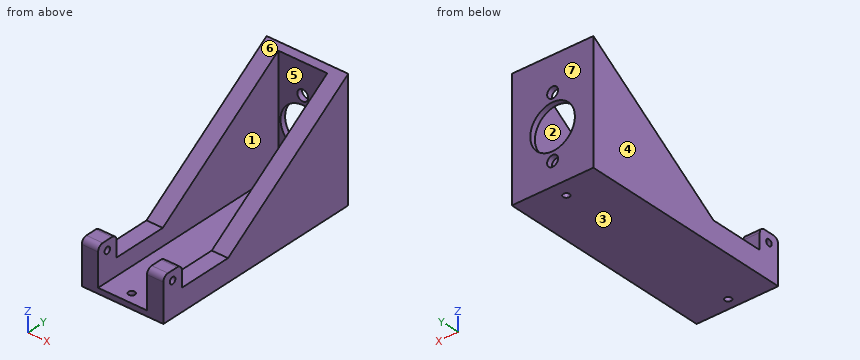
Solid Edge part; units mm, degrees
sketch "Sketch1" plane through (0, 0, 0) normal (0, -1, 0) x (1, 0, 0)
  line L0 (0, 110) -> (0, 0)
  line L1 (0, 0) -> (75, 0)
  line L2 (75, 0) -> (75, 110)
  line L3 (75, 110) -> (0, 110)
  dimension "D1" = 75
extrude "Protrusion1" add sketch "Sketch1" against normal blind 200
sketch "Sketch2" plane through (37.5, 0, 62.5) normal (0, -1, 0) x (1, 0, 0)
  line L0 (-22.5, 47.5) -> (-22.5, -57.5)
  line L1 (-22.5, -57.5) -> (22.5, -57.5)
  line L2 (22.5, -57.5) -> (22.5, 47.5)
  dimension "D1" = 22.5
extrude "ExtrudedCutout_1" cut sketch "Sketch2" against normal blind 195 material side at (15.05, 0, 57.5)
sketch "Sketch3" plane through (0, 100, 62.5) normal (-1, 0, 0) x (0, -1, 0)
  line L0 (-100, 47.5) -> (30, -42.1258)
  line L1 (30, -42.1258) -> (80, -42.1258)
  line L2 (80, -42.1258) -> (80, -22.5)
  line L3 (80, -22.5) -> (100, -22.5)
  line L4 (100, 47.5) -> (100, -22.5)
  line L5 (-100, 47.5) -> (100, 47.5)
  dimension "D1" = 80
  dimension "D2" = 30
  dimension "D3" = 100
extrude "ExtrudedCutout_2" cut sketch "Sketch3" against normal blind 140
hole "hål_till_pedal_vänster" at (0, 10, 31.4) direction (1, 0, 0) diameter 6 end up to next
hole "Hål_till_pedal_höger_" at (75, 10, 31.4) direction (-1, 0, 0) diameter 6 end up to next
fillet "Avrundning" radius 5 4 edges at (67.5, 0, 40) (67.5, 20, 40) (7.5, 0, 40) (7.5, 20, 40)
hole "Hål_till_huvudcylinder" at (37.5, 200, 50) direction (0, -1, 0) diameter 41 end up to next
hole "Hole1" at (37.5, 200, 78.6) direction (0, -1, 0) diameter 10 end up to next
hole "Hole2" at (37.5, 200, 21.4) direction (0, -1, 0) diameter 10 end up to next
hole "Hole3" at (37.5, 10, 5) direction (0, 0, -1) diameter 6 end through all
hole "Hole4" at (37.5, 185, 5) direction (0, 0, -1) diameter 6 end through all
properties material "Aluminum, 1060"
Geometry: final body of the model. Coordinates: model frame, mm. Face numbers are marked on the shaded views. A direction names the side the tool comes from. Coordinates: 2 decimals unless noted, no trailing zeros. Order: outer loops, then holes, each group sorted by start corner. A loop starts at its lowest first (then second) coordinate and runs counter-clockwise, first axis right, second up. Notation, with made-up numbers: M 46.5,44 L 97.5,44 A9 cw 97.5,50 Z; hole C 28.5,30.25 d4. An arc over 180 degrees is marked long. Answer in a Markdown table with one row per item. Add a question column.
Q1. Mould query, pull axis X, two halves, no side actions, for the marked faces 1, 2, 3 and 4. Classes: released by +X, released by -X, zero draft, split by the parting line, or undercut.
Q2. Line query: L1, parallel to Y at x = 37, z = 2; L2, parallel to Z at x = 65, y = 10; L3, parallel to X at y = 160, z = 37. Output: solid intervals per line, ascending.
Q3. Section query B-B on x = 64. Return the cut outline in (y, z).
Q4. Reachability of the marked faces 5, 6 and 7 from +Z, -Z, +X, -X, +Y, -Y: full face, straight path, thin tool, end or side. Return the list, or none.
Q5. Contact query for flat-ended pins moving along their axis: P1, Ø12, axis at y = 74, z = 29.5, coming from the +X side; P2, Ø12, axis at x = 67.5, y = 34, coming from the +Z side; P3, Ø5, axis at x = 4.5, y = 8.5, coming from the +Z side; P4, Ø22.5, axis at x = 29, y = 86.5, coming from the +Z side. Output: stop coordinate, or through.
Q6. Section query A-A on x = 37.5. Return the cut outline in (y, z), and give its area (3 significant figures).
Q7. Section query D-D on z = 45. Return the cut outline in (x, y), and give its area (3 significant figures).
Q8. Section query C-C on y = 10. Return the cut outline in (x, z).
Completed:
| question | item | result |
|---|---|---|
| 1 | face 1 | undercut |
| 1 | face 2 | undercut |
| 1 | face 3 | zero draft |
| 1 | face 4 | released by -X |
| 2 | L1 | y = 0 to 7.04, 12.96 to 182.04, 187.96 to 200 |
| 2 | L2 | z = 0 to 28.4, 34.4 to 40 |
| 2 | L3 | x = 0 to 15, 60 to 75 |
| 3 | outline | M 0,0 L 200,0 L 200,110 L 70,20.37 L 20,20.37 L 20,35 A5 ccw 15,40 L 5,40 A5 ccw 0,35 Z; hole C 10,31.4 d6 |
| 4 | face 5 | +Z, -Y |
| 4 | face 6 | +Z, +X, -X |
| 4 | face 7 | +Z, -Z, +X, -X, +Y |
| 5 | P1 | stops at x = 75 |
| 5 | P2 | stops at z = 20.37 |
| 5 | P3 | stops at z = 40 |
| 5 | P4 | stops at z = 5 |
| 6 | outline | M 0,0 L 7,0 L 7,5 L 0,5 Z; M 13,0 L 182,0 L 182,5 L 13,5 Z; M 188,0 L 200,0 L 200,16.4 L 195,16.4 L 195,5 L 188,5 Z; M 195,26.4 L 200,26.4 L 200,29.5 L 195,29.5 Z; M 195,70.5 L 200,70.5 L 200,73.6 L 195,73.6 Z; M 195,83.6 L 200,83.6 L 200,110 L 195,106.55 Z |
| 6 | area | 1,150 mm2 |
| 7 | outline | M 0,105.72 L 15,105.72 L 15,195 L 17.62,195 L 17.62,200 L 0,200 Z; M 57.38,195 L 60,195 L 60,105.72 L 75,105.72 L 75,200 L 57.38,200 Z |
| 7 | area | 2,850 mm2 |
| 8 | outline | M 0,0 L 34.5,0 L 34.5,5 L 15,5 L 15,28.4 L 0,28.4 Z; M 0,34.4 L 15,34.4 L 15,40 L 0,40 Z; M 40.5,0 L 75,0 L 75,28.4 L 60,28.4 L 60,5 L 40.5,5 Z; M 60,34.4 L 75,34.4 L 75,40 L 60,40 Z |
